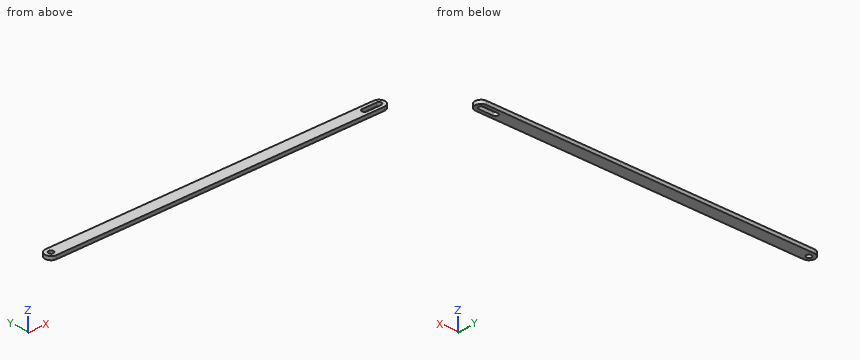
from build123d import *

# Parameters (mm, degrees)
SKETCH_1_R      = 1.7
EXTRUDE_1_DEPTH = 2.4


with BuildPart() as part:
    # 草图1 → 凸台-拉伸1 (new body)
    with BuildSketch(Plane.XY):
        with BuildLine():
            Line((-53.850242828, -4), (166.149757172, -4))
            ThreePointArc((166.149757172, -4), (170.149757172, 0), (166.149757172, 4))
            Line((166.149757172, 4), (-53.850242828, 4))
            ThreePointArc((-53.850242828, 4), (-57.850242828, 0), (-53.850242828, -4))
        make_face()
        with Locations((-53.850242828, 0)):
            Circle(SKETCH_1_R, mode=Mode.SUBTRACT)
        with BuildLine():
            ThreePointArc((156.438691487, 1.7), (154.738691487, 0), (156.438691487, -1.7))
            Line((156.438691487, -1.7), (166.149757172, -1.7))
            ThreePointArc((166.149757172, -1.7), (167.849757172, 0), (166.149757172, 1.7))
            Line((166.149757172, 1.7), (156.438691487, 1.7))
        make_face(mode=Mode.SUBTRACT)
    extrude(amount=EXTRUDE_1_DEPTH)


solid = part.part
Here's how the part is built. I have some questions about the finished solid (model axes, mm). Coordinates: 2 decimals unless noted, no trailing zeros. Write each loop counter-clockwise with the first axis right and the second up, starting at its lowest first coordinate (ties: lowest second). Pieces come first, ordered by that corner, then holes.
1) If I drill on line 1 (X direction, y = -0.75, z = 0.85); line 2 (X direction, y = 0.5, z = 0.95); line 3 (Y direction, x = 155.5, z = 1.85), over which ranges is the centre line in solid material (lowest first)?
Filled in:
line 1: x = -57.78 to -55.38, -52.32 to 154.91, 167.68 to 170.08
line 2: x = -57.82 to -55.48, -52.23 to 154.81, 167.77 to 170.12
line 3: y = -4 to -1.42, 1.42 to 4
2) If we section it at A-A (y = 0): List the corners of the cut face in (x, z) for me, plus the area to 3 significant figures.
Filled in:
outline: (-57.85, 0) - (-55.55, 0) - (-55.55, 2.4) - (-57.85, 2.4) - close; (-52.15, 0) - (154.74, 0) - (154.74, 2.4) - (-52.15, 2.4) - close; (167.85, 0) - (170.15, 0) - (170.15, 2.4) - (167.85, 2.4) - close
area: 508 mm2
3) If we section it at B-B (z = 1.7): List the corners of the cut face in (x, y) for me.
Filled in:
outline: (-53.85, -4) - (166.15, -4) arc R4 ccw to (166.15, 4) - (-53.85, 4) arc R4 ccw to start; hole circle Ø3.4 at (-53.85, 0); hole (156.44, -1.7) - (166.15, -1.7) arc R1.7 ccw to (166.15, 1.7) - (156.44, 1.7) arc R1.7 ccw to start
